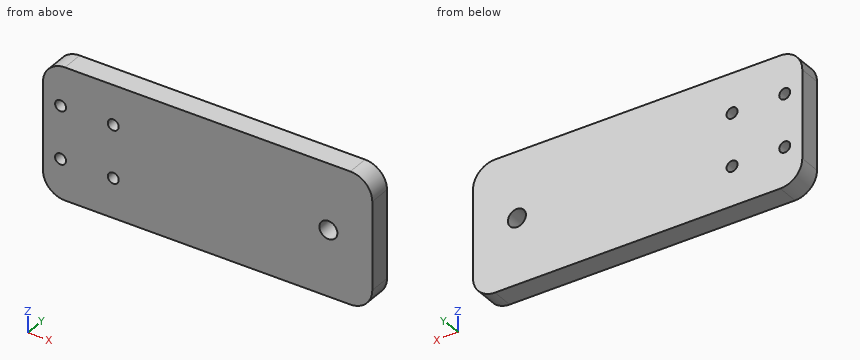
from build123d import *

# Parameters (mm, degrees)
SKETCH_1_W          = 150
SKETCH_1_H          = 60
EXTRUDE_1_DEPTH     = 10
FILLET_1_R          = 10
SKETCH_2_R          = 2.5
SKETCH_2_R_2        = 4.1
CUT_EXTRUDE_1_DEPTH = 82.39410298


with BuildPart() as part:
    # ｽｹｯﾁ1 → ﾎﾞｽ - 押し出し1 (new body)
    with BuildSketch(Plane(origin=(0, 0, 0), x_dir=(1, 0, 0), z_dir=(0, 1, 0))):
        Rectangle(SKETCH_1_W, SKETCH_1_H)
    extrude(amount=EXTRUDE_1_DEPTH)

    # ﾌｨﾚｯﾄ1
    fillet_1_edges = [part.edges().sort_by_distance(p)[0] for p in [
        (75, 5, 30),
        (-75, 5, 30),
        (-75, 5, -30),
        (75, 5, -30),
    ]]
    fillet(fillet_1_edges, radius=FILLET_1_R)

    # ｽｹｯﾁ2 → ｶｯﾄ - 押し出し1 (cut, through all)
    with BuildSketch(Plane(origin=(0, 10, 0), x_dir=(1, 0, 0), z_dir=(0, 1, 0))):
        with Locations(Location((-67, 12, 0), (0, 0, 270))):
            Circle(SKETCH_2_R)
        with Locations(Location((-43, 12, 0), (0, 0, 270))):
            Circle(SKETCH_2_R)
        with Locations(Location((-67, -12, 0), (0, 0, 270))):
            Circle(SKETCH_2_R)
        with Locations(Location((-43, -12, 0), (0, 0, 270))):
            Circle(SKETCH_2_R)
        with Locations(Location((55, 0, 0), (0, 0, 270))):
            Circle(SKETCH_2_R_2)
    extrude(amount=-CUT_EXTRUDE_1_DEPTH, mode=Mode.SUBTRACT)


solid = part.part
Design review of the part built by this model. Coordinates are the model's own, in mm. Coordinates: 2 decimals unless noted, no trailing zeros. Order: outer loops, then holes, each group sorted by start corner. A loop starts at its lowest first (then second) coordinate and runs counter-clockwise, first axis right, second up. Notation, with made-up numbers: (-36, 89.25) -> (-31, 89.25) arc R25 ccw to (-31, 126.25) -> close; hole circle Ø6 at (35.25, 76.5). An arc over 180 degrees is marked (long way). One line per item, written item: value.
1) We need section A-A, the plane x = 55. Give the boundary of the cut face in (y, z).
Output values:
outline: (0, -30) -> (10, -30) -> (10, -4.1) -> (0, -4.1) -> close; (0, 4.1) -> (10, 4.1) -> (10, 30) -> (0, 30) -> close
2) We need section D-D, the plane x = -67. Give the boundary of the cut face in (y, z), then the cut area to 3 significant figures.
Output values:
outline: (0, -29.8) -> (10, -29.8) -> (10, -14.5) -> (0, -14.5) -> close; (0, -9.5) -> (10, -9.5) -> (10, 9.5) -> (0, 9.5) -> close; (0, 14.5) -> (10, 14.5) -> (10, 29.8) -> (0, 29.8) -> close
area: 496 mm2
3) We need section B-B, the plane z = 0. Give the boundary of the cut face in (x, y).
Output values:
outline: (-75, 0) -> (50.9, 0) -> (50.9, 10) -> (-75, 10) -> close; (59.1, 0) -> (75, 0) -> (75, 10) -> (59.1, 10) -> close
4) To check wall thickness, follow probe 1 along X at (y, z) = (4, 12); probe 2 along X at (y, z) = (4.5, 0); probe 3 along X at (y, z) = (4.25, 3.5). State the ranges of each line that lie inside material, in increasing order. Write a range as [from, to].
Output values:
probe 1: x = [-75, -69.5], [-64.5, -45.5], [-40.5, 75]
probe 2: x = [-75, 50.9], [59.1, 75]
probe 3: x = [-75, 52.86], [57.14, 75]
5) Clearance check with flat-ended pins moving along their axes: P1, Ø8, axis at x = -67, z = 12, coming from the +Y side; P2, Ø3, axis at x = -43, z = 12, coming from the +Y side. State where each tip first meets the part, or that it passes through.
Output values:
P1: stops at y = 10
P2: passes through
6) We need section C-C, the plane y = 7.5. Give the boundary of the cut face in (x, z).
Output values:
outline: (-75, -20) arc R10 ccw to (-65, -30) -> (65, -30) arc R10 ccw to (75, -20) -> (75, 20) arc R10 ccw to (65, 30) -> (-65, 30) arc R10 ccw to (-75, 20) -> close; hole circle Ø5 at (-67, -12); hole circle Ø5 at (-67, 12); hole circle Ø5 at (-43, -12); hole circle Ø5 at (-43, 12); hole circle Ø8.2 at (55, 0)
